The model under review builds one solid part; all positions refer to its coordinate system, in mm. A direction names the side the tool comes from. Coordinates: 2 decimals unless noted, no trailing zeros. Write each loop counter-clockwise with the first axis right and the second up, starting at its lowest first coordinate (ties: lowest second). Pieces come first, ordered by that corner, then holes.
```python
from build123d import *


with BuildPart() as f1:
    # F0 (on Front) → F1 (revolve)
    with BuildSketch(Plane.XZ):
        with BuildLine():
            Line((0, 50.8), (0, 0))
            Line((0, 0), (10.261248, 0))
            Line((10.261248, 0), (21.929258, 7.154912))
            ThreePointArc((21.929258, 7.154912), (24.1506, 9.46627), (24.959791, 12.568196))
            Line((24.959791, 12.568196), (24.959791, 17.333189))
            Line((24.959791, 17.333189), (10.261248, 17.333189))
            Line((10.261248, 17.333189), (10.261248, 50.8))
            Line((10.261248, 50.8), (0, 50.8))
        make_face()
    revolve(axis=Axis((0, 0, 25.4), (0, 0, 1)))


solid = f1.part
```
Item 1: Take a section at D-D, the plane z = 11. Write out the cut boundary in (x, y), plus the area to 3 significant figures.
Solved:
outline: circle Ø49.53 at (0, 0)
area: 1,930 mm2
Item 2: To check wall thickness, follow line 1 along Y through (x, z) = (7.5, 39.5); line 2 along X through (y, z) = (-9.5, 9); line 3 along Y through (x, z) = (-9, 7). State the ranges of each line that lie inside material, in increasing order.
Solved:
line 1: y = -7 to 7
line 2: x = -21.89 to 21.89
line 3: y = -19.72 to 19.72
Item 3: For pin 1 (5 mm diameter, centred on y = 3, z = 35.5, fed in from +X); pin 2 (6 mm diameter, centred on y = -0.5, z = 37, fed in from +X); pin 3 (1.5 mm diameter, centred on x = -8, y = 10, fed in from +Z), all flat-tipped, find the tip position at first contact; note any pin that passes through.
Solved:
pin 1: stops at x = 10.25
pin 2: stops at x = 10.26
pin 3: stops at z = 17.33
Item 4: Take a section at C-C, the plane z = 19.5. Write out the cut boundary in (x, y), plus the area to 3 significant figures.
Solved:
outline: circle Ø20.52 at (0, 0)
area: 331 mm2
Item 5: Take a section at A-A, the plane y = 0. Write out the cut boundary in (x, z), plus the area to 3 significant figures.
Solved:
outline: (-24.96, 12.57) arc R6.35 ccw to (-21.93, 7.15) - (-10.26, 0) - (10.26, 0) - (21.93, 7.15) arc R6.35 ccw to (24.96, 12.57) - (24.96, 17.33) - (10.26, 17.33) - (10.26, 50.8) - (-10.26, 50.8) - (-10.26, 17.33) - (-24.96, 17.33) - close
area: 1,420 mm2
Item 6: Machinability: for faces 1 (the face through (0, 0, 0)), 2 (the face through (-8.143, -6.244, 34.301)), which of the approach directions +Z, -Z, +X, -X, +Y, -Y give a long, thin tool a straight path to every point of the face, cutting with its end or side? Answer none if there is none.
Solved:
face 1: -Z, +X, -X, +Y, -Y
face 2: +Z
